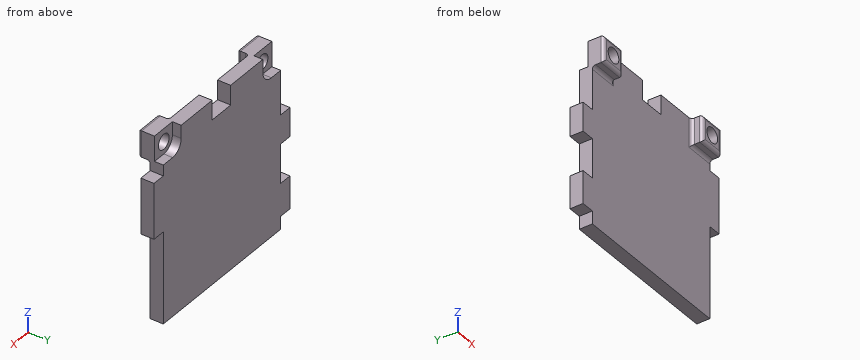
from build123d import *

# Parameters (mm, degrees)
SKETCH_1_W               = 25.25
SKETCH_1_H               = 26
EXTRUDE_1_DEPTH          = 2
SKETCH_3_W               = 4
SKETCH_3_H               = 4
EXTRUDE_2_DEPTH          = 1.8
CUT_EXTRUDE_2_DEPTH      = 2
CUT_EXTRUDE_2_DEPTH_BACK = 1.8
SKETCH_4_R               = 1.15
SKETCH_5_R               = 1.85
CUT_EXTRUDE_3_DEPTH      = 1.35
SKETCH_7_W               = 25.25
SKETCH_7_H               = 2
EXTRUDE_4_DEPTH          = 2
FILLET_3_R               = 0.5
SKETCH_8_W               = 8.5
SKETCH_8_H               = 2
EXTRUDE_5_DEPTH          = 2
SKETCH_9_W               = 5
SKETCH_9_H               = 2
EXTRUDE_6_DEPTH          = 2
SKETCH_10_W              = 4.4
SKETCH_10_H              = 2
EXTRUDE_7_DEPTH          = 2
SKETCH_11_W              = 4
SKETCH_11_H              = 3
CUT_EXTRUDE_4_DEPTH      = 2
CUT_EXTRUDE_5_DEPTH      = 1.35


with BuildPart() as part:
    # 草图1 → 凸台-拉伸1 (new body)
    with BuildSketch(Plane(origin=(0, 0, 0), x_dir=(1, 0, 0), z_dir=(0, 1, 0))):
        Rectangle(SKETCH_1_W, SKETCH_1_H)
    extrude(amount=EXTRUDE_1_DEPTH)

    # 草图3 → 凸台-拉伸2 (add)
    with BuildSketch(Plane(origin=(0, 0, 0), x_dir=(1, 0, 0), z_dir=(0, 1, 0))):
        with Locations((-10.625, -11)):
            Rectangle(SKETCH_3_W, SKETCH_3_H)
        with Locations((10.625, -11)):
            Rectangle(SKETCH_3_W, SKETCH_3_H)
    extrude(amount=-EXTRUDE_2_DEPTH)

    # 草图4 → 切除-拉伸2 (cut, two sides: drawn at the far end of the back side and taken through both)
    with BuildSketch(Plane(origin=(0, 0, 0), x_dir=(1, 0, 0), z_dir=(0, 1, 0)).offset(-CUT_EXTRUDE_2_DEPTH_BACK)):
        with Locations(Location((-10.625, -11, 0), (0, 0, 270))):
            Circle(SKETCH_4_R)
        with Locations(Location((10.625, -11, 0), (0, 0, 90))):
            Circle(SKETCH_4_R)
    extrude(amount=CUT_EXTRUDE_2_DEPTH + CUT_EXTRUDE_2_DEPTH_BACK, mode=Mode.SUBTRACT)

    # 草图5 → 切除-拉伸3 (cut)
    with BuildSketch(Plane(origin=(0, 2, 0), x_dir=(1, 0, 0), z_dir=(0, 1, 0))):
        with Locations(Location((-10.625, -11, 0), (0, 0, 270))):
            Circle(SKETCH_5_R)
        with Locations(Location((10.625, -11, 0), (0, 0, 270))):
            Circle(SKETCH_5_R)
    extrude(amount=-CUT_EXTRUDE_3_DEPTH, mode=Mode.SUBTRACT)

    # 草图7 → 凸台-拉伸4 (add)
    with BuildSketch(Plane(origin=(0, 0, -13), x_dir=(-1, 0, 0), z_dir=(0, 0, -1))):
        with Locations((0, 1)):
            Rectangle(SKETCH_7_W, SKETCH_7_H)
    extrude(amount=EXTRUDE_4_DEPTH)

    # 圆角3
    fillet_3_edges = [part.edges().sort_by_distance(p)[0] for p in [
        (-12.625, -1.8, 11),
        (-10.625, -1.8, 9),
        (-8.625, -1.8, 11),
        (-10.625, -1.8, 13),
        (-8.625, 0, 11),
        (-10.625, 0, 9),
        (12.625, -1.8, 11),
        (10.625, -1.8, 13),
        (8.625, -1.8, 11),
        (10.625, -1.8, 9),
        (10.625, 0, 9),
        (8.625, 0, 11),
    ]]
    fillet(fillet_3_edges, radius=FILLET_3_R)

    # 草图8 → 凸台-拉伸5 (add)
    with BuildSketch(Plane(origin=(12.625, 0, 0), x_dir=(0, 0, -1), z_dir=(1, 0, 0))):
        with Locations((-3.25, 1)):
            Rectangle(SKETCH_8_W, SKETCH_8_H)
    extrude(amount=EXTRUDE_5_DEPTH)

    # 草图9 → 凸台-拉伸6 (add)
    with BuildSketch(Plane.ZY.offset(12.625)):
        with Locations((-10.530736821, 1)):
            Rectangle(SKETCH_9_W, SKETCH_9_H)
    extrude(amount=EXTRUDE_6_DEPTH)

    # 草图10 → 凸台-拉伸7 (add)
    with BuildSketch(Plane.ZY.offset(12.625)):
        with Locations((0.16, 1)):
            Rectangle(SKETCH_10_W, SKETCH_10_H)
    extrude(amount=EXTRUDE_7_DEPTH)

    # 草图11 → 切除-拉伸4 (cut)
    with BuildSketch(Plane(origin=(0, 2, 0), x_dir=(1, 0, 0), z_dir=(0, 1, 0))):
        with Locations((0.125, -11.5)):
            Rectangle(SKETCH_11_W, SKETCH_11_H)
    extrude(amount=-CUT_EXTRUDE_4_DEPTH, mode=Mode.SUBTRACT)

    # 草图12 → 切除-拉伸5 (cut)
    with BuildSketch(Plane(origin=(0, 2, 0), x_dir=(1, 0, 0), z_dir=(0, 1, 0))):
        Polygon((-10.625, -9.15), (-12.625, -9.15), (-12.625, -13), (-8.775, -13), (-8.775, -11), align=None)
        Polygon((8.775, -11), (10.625, -9.15), (12.625, -9.15), (12.625, -13), (8.775, -13), align=None)
    extrude(amount=-CUT_EXTRUDE_5_DEPTH, mode=Mode.SUBTRACT)


solid = part.part
Geometry: final body of the model. Coordinates: model frame, mm. Give positions to 0.01 mm unless a question says otherwise; leave off trailing zeros. Write each loop counter-clockwise with the first axis right and the second up, starting at its lowest first coordinate (ties: lowest second). Pieces come first, ordered by that corner, then holes.
(1) Cut plane D-D, the plane z = 6.5. Return loops of the section in (x, y) (3 decimals), then the cut area to 3 significant figures.
(2) Cut plane A-A, the plane y = 1.65. Return loops of the section in (x, z) (3 decimals), then the cut area to 3 significant figures.
(3) Ray query, line 1 (X direction, y = -0.55, z = 11) (3 decimals); line 2 (Y direction, x = -5.75, z = -11); line 3 (X direction, y = 1.5, z = 8.75) (3 decimals). Return the intervals inside material, ascending.
(4) Cut plane C-C, the plane x = 1. Return loops of the section in (y, z), then the cut area to 3 significant figures.
(5) Cut plane B-B, the plane x = 10. Return loops of the section in (y, z), then the cut area to 3 significant figures.
(6) First-contact query: P1, Ø3.5, axis at x = 10.625, z = 11, coming from the +Y side; P2, Ø2, axis at y = 0.5, z = -9, coming from the +X side (3 decimals); P3, Ø2, axis at x = -14, y = 0.5, coming from the +Z side. Flat tips, straight axial feed; report the tip coordinate or a pass-through.
Values follow:
1. outline: (-12.625, 0) - (14.625, 0) - (14.625, 2) - (-12.625, 2) - close
1. area: 54.5 mm2
2. outline: (-14.625, -13.031) - (-12.625, -13.031) - (-12.625, -15) - (12.625, -15) - (12.625, -1) - (14.625, -1) - (14.625, 7.5) - (12.625, 7.5) - (12.625, 9.15) - (10.625, 9.15) arc R1.85 cw to (8.775, 11) - (8.775, 13) - (2.125, 13) - (2.125, 10) - (-1.875, 10) - (-1.875, 13) - (-8.775, 13) - (-8.775, 11) arc R1.85 cw to (-10.625, 9.15) - (-12.625, 9.15) - (-12.625, 2.36) - (-14.625, 2.36) - (-14.625, -2.04) - (-12.625, -2.04) - (-12.625, -8.031) - (-14.625, -8.031) - close
2. area: 703 mm2
3. line 1: x = -12.625 to -11.775, -9.475 to -8.625, 8.625 to 9.475, 11.775 to 12.625
3. line 2: y = 0 to 2
3. line 3: x = -12.625 to 12.625
4. outline: (0, -15) - (2, -15) - (2, 10) - (0, 10) - close
4. area: 50.0 mm2
5. outline: (-1.8, 9.5) arc R0.5 ccw to (-1.3, 9) - (-0.5, 9) arc R0.5 cw to (0, 8.5) - (0, -15) - (2, -15) - (2, 9.26) - (0.65, 9.26) - (0.65, 10.03) - (-1.8, 10.03) - close; (-1.8, 11.97) - (0.65, 11.97) - (0.65, 13) - (-1.3, 13) arc R0.5 ccw to (-1.8, 12.5) - close
5. area: 53.4 mm2
6. P1: stops at y = 0.65
6. P2: stops at x = 12.625
6. P3: stops at z = 2.36
